from build123d import *

# Parameters (mm, degrees)
F0_R     = 1.778
F1_DEPTH = 5.08
F2_R     = 3.81
F2_R_2   = 1.778
F3_DEPTH = 6.35
F4_R     = 5.08
F5_R     = 1.016


with BuildPart() as f1:
    # F0 (on Front) → F1 (new body)
    with BuildSketch(Plane.XZ):
        with BuildLine():
            ThreePointArc((7.605604, -0.468175), (7.6164, -0.234198), (7.62, 0))
            ThreePointArc((7.62, 0), (7.6164, 0.234198), (7.605604, 0.468175))
            ThreePointArc((7.605604, 0.468175), (7.247051, 2.354709), (6.428249, 4.0917))
            ThreePointArc((6.428249, 4.0917), (6.164709, 4.478924), (5.877877, 4.849223))
            ThreePointArc((5.877877, 4.849223), (4.478924, 6.164709), (2.795522, 7.088685))
            ThreePointArc((2.795522, 7.088685), (2.354709, 7.247051), (1.905, 7.378033))
            ThreePointArc((1.905, 7.378033), (0, 7.62), (-1.905, 7.378033))
            ThreePointArc((-1.905, 7.378033), (-2.354709, 7.247051), (-2.795522, 7.088685))
            ThreePointArc((-2.795522, 7.088685), (-4.478924, 6.164709), (-5.877877, 4.849223))
            ThreePointArc((-5.877877, 4.849223), (-6.164709, 4.478924), (-6.428249, 4.0917))
            ThreePointArc((-6.428249, 4.0917), (-7.247051, 2.354709), (-7.605604, 0.468175))
            ThreePointArc((-7.605604, 0.468175), (-7.62, 0), (-7.605604, -0.468175))
            ThreePointArc((-7.605604, -0.468175), (-7.247051, -2.354709), (-6.428249, -4.0917))
            ThreePointArc((-6.428249, -4.0917), (-6.164709, -4.478924), (-5.877877, -4.849223))
            ThreePointArc((-5.877877, -4.849223), (-4.478924, -6.164709), (-2.795522, -7.088685))
            ThreePointArc((-2.795522, -7.088685), (-2.354709, -7.247051), (-1.905, -7.378033))
            ThreePointArc((-1.905, -7.378033), (0, -7.62), (1.905, -7.378033))
            ThreePointArc((1.905, -7.378033), (2.354709, -7.247051), (2.795522, -7.088685))
            ThreePointArc((2.795522, -7.088685), (4.478924, -6.164709), (5.877877, -4.849223))
            ThreePointArc((5.877877, -4.849223), (6.164709, -4.478924), (6.428249, -4.0917))
            ThreePointArc((6.428249, -4.0917), (7.247051, -2.354709), (7.605604, -0.468175))
        make_face()
        Circle(F0_R, mode=Mode.SUBTRACT)
        with BuildLine():
            ThreePointArc((6.428249, 4.0917), (7.247051, 2.354709), (7.605604, 0.468175))
            Line((7.605604, 0.468175), (9.689785, 1.412438))
            Line((9.689785, 1.412438), (11.830752, 3.04283))
            Line((11.830752, 3.04283), (11.35981, 4.49224))
            Line((11.35981, 4.49224), (8.66941, 4.552826))
            Line((8.66941, 4.552826), (6.428249, 4.0917))
        make_face()
        with BuildLine():
            Line((9.689785, -1.412438), (7.605604, -0.468175))
            ThreePointArc((7.605604, -0.468175), (7.247051, -2.354709), (6.428249, -4.0917))
            Line((6.428249, -4.0917), (8.66941, -4.552826))
            Line((8.66941, -4.552826), (11.35981, -4.49224))
            Line((11.35981, -4.49224), (11.830752, -3.04283))
            Line((11.830752, -3.04283), (9.689785, -1.412438))
        make_face()
        with BuildLine():
            ThreePointArc((2.795522, 7.088685), (4.478924, 6.164709), (5.877877, 4.849223))
            Line((5.877877, 4.849223), (7.00899, 6.838199))
            Line((7.00899, 6.838199), (7.782749, 9.415643))
            Line((7.782749, 9.415643), (6.549807, 10.311428))
            Line((6.549807, 10.311428), (4.337616, 8.779065))
            Line((4.337616, 8.779065), (2.795522, 7.088685))
        make_face()
        with BuildLine():
            Line((7.00899, -6.838199), (5.877877, -4.849223))
            ThreePointArc((5.877877, -4.849223), (4.478924, -6.164709), (2.795522, -7.088685))
            Line((2.795522, -7.088685), (4.337616, -8.779065))
            Line((4.337616, -8.779065), (6.549807, -10.311428))
            Line((6.549807, -10.311428), (7.782749, -9.415643))
            Line((7.782749, -9.415643), (7.00899, -6.838199))
        make_face()
        with BuildLine():
            ThreePointArc((-1.905, 7.378033), (0, 7.62), (1.905, 7.378033))
            Line((1.905, 7.378033), (1.651, 9.652))
            Line((1.651, 9.652), (0.762, 12.192))
            Line((0.762, 12.192), (-0.762, 12.192))
            Line((-0.762, 12.192), (-1.651, 9.652))
            Line((-1.651, 9.652), (-1.905, 7.378033))
        make_face()
        with BuildLine():
            Line((1.651, -9.652), (1.905, -7.378033))
            ThreePointArc((1.905, -7.378033), (0, -7.62), (-1.905, -7.378033))
            Line((-1.905, -7.378033), (-1.651, -9.652))
            Line((-1.651, -9.652), (-0.762, -12.192))
            Line((-0.762, -12.192), (0.762, -12.192))
            Line((0.762, -12.192), (1.651, -9.652))
        make_face()
        with BuildLine():
            ThreePointArc((-5.877877, 4.849223), (-4.478924, 6.164709), (-2.795522, 7.088685))
            Line((-2.795522, 7.088685), (-4.337616, 8.779065))
            Line((-4.337616, 8.779065), (-6.549807, 10.311428))
            Line((-6.549807, 10.311428), (-7.782749, 9.415643))
            Line((-7.782749, 9.415643), (-7.00899, 6.838199))
            Line((-7.00899, 6.838199), (-5.877877, 4.849223))
        make_face()
        with BuildLine():
            Line((-4.337616, -8.779065), (-2.795522, -7.088685))
            ThreePointArc((-2.795522, -7.088685), (-4.478924, -6.164709), (-5.877877, -4.849223))
            Line((-5.877877, -4.849223), (-7.00899, -6.838199))
            Line((-7.00899, -6.838199), (-7.782749, -9.415643))
            Line((-7.782749, -9.415643), (-6.549807, -10.311428))
            Line((-6.549807, -10.311428), (-4.337616, -8.779065))
        make_face()
        with BuildLine():
            ThreePointArc((-7.605604, 0.468175), (-7.247051, 2.354709), (-6.428249, 4.0917))
            Line((-6.428249, 4.0917), (-8.66941, 4.552826))
            Line((-8.66941, 4.552826), (-11.35981, 4.49224))
            Line((-11.35981, 4.49224), (-11.830752, 3.04283))
            Line((-11.830752, 3.04283), (-9.689785, 1.412438))
            Line((-9.689785, 1.412438), (-7.605604, 0.468175))
        make_face()
        with BuildLine():
            Line((-8.66941, -4.552826), (-6.428249, -4.0917))
            ThreePointArc((-6.428249, -4.0917), (-7.247051, -2.354709), (-7.605604, -0.468175))
            Line((-7.605604, -0.468175), (-9.689785, -1.412438))
            Line((-9.689785, -1.412438), (-11.830752, -3.04283))
            Line((-11.830752, -3.04283), (-11.35981, -4.49224))
            Line((-11.35981, -4.49224), (-8.66941, -4.552826))
        make_face()
    extrude(amount=F1_DEPTH)

    # F2 (on face) → F3 (join)
    with BuildSketch(Plane.XZ.offset(5.08)):
        Circle(F2_R)
        Circle(F2_R_2, mode=Mode.SUBTRACT)
    extrude(amount=F3_DEPTH)

    # F4
    f4_edges = [f1.edges().sort_by_distance(p)[0] for p in [
        (7.00899, -2.54, 6.838199),
        (4.337616, -2.54, 8.779065),
        (1.651, -2.54, 9.652),
        (-4.337616, -2.54, 8.779065),
        (-8.66941, -2.54, 4.552826),
        (-9.689785, -2.54, -1.412438),
        (-7.00899, -2.54, -6.838199),
        (-1.651, -2.54, -9.652),
        (4.337616, -2.54, -8.779065),
        (8.66941, -2.54, -4.552826),
        (9.689785, -2.54, 1.412438),
        (9.689785, -2.54, -1.412438),
        (8.66941, -2.54, 4.552826),
        (-1.651, -2.54, 9.652),
        (-7.00899, -2.54, 6.838199),
        (-9.689785, -2.54, 1.412438),
        (-8.66941, -2.54, -4.552826),
        (-4.337616, -2.54, -8.779065),
        (1.651, -2.54, -9.652),
        (7.00899, -2.54, -6.838199),
    ]]
    fillet(f4_edges, radius=F4_R)

    # F5
    f5_edges = [f1.edges().sort_by_distance(p)[0] for p in [
        (0.762, -2.54, 12.192),
        (-0.762, -2.54, 12.192),
        (-6.549807, -2.54, 10.311428),
        (-7.782749, -2.54, 9.415643),
        (-11.35981, -2.54, 4.49224),
        (6.549807, -2.54, 10.311428),
        (7.782749, -2.54, 9.415643),
        (11.35981, -2.54, 4.49224),
        (-11.830752, -2.54, 3.04283),
        (-11.830752, -2.54, -3.04283),
        (-11.35981, -2.54, -4.49224),
        (-7.782749, -2.54, -9.415643),
        (-6.549807, -2.54, -10.311428),
        (-0.762, -2.54, -12.192),
        (0.762, -2.54, -12.192),
        (6.549807, -2.54, -10.311428),
        (7.782749, -2.54, -9.415643),
        (11.830752, -2.54, -3.04283),
        (11.35981, -2.54, -4.49224),
        (11.830752, -2.54, 3.04283),
    ]]
    fillet(f5_edges, radius=F5_R)


solid = f1.part
Here's how the part is built. I have some questions about the finished solid (model axes, mm). A direction names the side the tool comes from. Coordinates: 2 decimals unless noted, no trailing zeros. Write each loop counter-clockwise with the first axis right and the second up, starting at its lowest first coordinate (ties: lowest second). Pieces come first, ordered by that corner, then holes. Notation, with made-up numbers: (68, 74) - (110, 74) arc R23 cw to (110, 86) - close; hole circle Ø9 at (-3.5, 43). An arc over 180 degrees is marked (long way). Use one line per item in the form item = value.
1) Suppose I cut it at D-D, the plane x = -4.25. Write out the boundary of the cut face in (y, z).
Solved:
outline = (-5.08, -8.66) - (0, -8.66) - (0, 8.66) - (-5.08, 8.66) - close
2) I need wall thicknesses on line 1 (X direction, y = -4, z = 7.75); line 2 (Y direction, x = 5.5, z = -9); line 3 (Z direction, x = 0, y = -8.25). Which ranges of each line are inside material? Lowest first, please.
Solved:
line_1 = -7.28 to -3.4, -1.86 to 1.86, 3.4 to 7.28
line_2 = -5.08 to 0
line_3 = -3.81 to -1.78, 1.78 to 3.81
3) Suppose I cut it at A-A, the plane x = 9.75. Write out the boundary of the cut face in (y, z), plus the area to 3 significant figures.
Solved:
outline = (-5.08, -4.53) - (0, -4.53) - (0, -1.49) - (-5.08, -1.49) - close; (-5.08, 1.49) - (0, 1.49) - (0, 4.53) - (-5.08, 4.53) - close
area = 30.9 mm2
4) Suppose I cut it at B-B, the plane z = -7.75. Write out the boundary of the cut face in (x, y), plus the area to 3 significant figures.
Solved:
outline = (-7.28, -5.08) - (-3.4, -5.08) - (-3.4, 0) - (-7.28, 0) - close; (-1.86, -5.08) - (1.86, -5.08) - (1.86, 0) - (-1.86, 0) - close; (3.4, -5.08) - (7.28, -5.08) - (7.28, 0) - (3.4, 0) - close
area = 58.4 mm2
5) Suppose I cut it at C-C, the plane y = -9. Write out the boundary of the cut face in (x, z).
Solved:
outline = circle Ø7.62 at (0, 0); hole circle Ø3.56 at (0, 0)
6) I'm going to push flat-ended pins straight in: P1, Ø3, axis at y = -1, z = -6.5, coming from the -X side; P2, Ø2, axis at y = -1, z = 1.5, coming from the +X side; P3, Ø1, axis at y = -4, z = 8.5, coming from the -X side. Where does each tip first touch, or does it pass through?
Solved:
P1 = -7.36
P2 = 11.12
P3 = -7.62
7) On a 3-axis mill with a long thin cutter (end or side, diameter ignored), from which of +Z, -Z, +X, -X, +Y, -Y can I reach the whole of each face in a straight line? I mean faces 4 (the cylindrical face through (-4.365, -2.576, 8.76)), 5 (the flat face through (7.38, -2.5, -8.07)), 6 (the cylindrical face through (-4.353, -2.576, -8.749)). Say none if no direction works.
Solved:
face_4 = +Z, +Y, -Y
face_5 = +X, +Y, -Y
face_6 = -Z, +Y, -Y
8) Thinking about a two-plate mould opening in X: for faces 1 (the flat face through (-7.279, -2.504, -4.267)), 2 (the flat face through (7.372, -2.504, 8.048)), 3 (the flat face through (-3, -5.08, 3)), which applies, released by +X, released by -X, zero draft, split by the parting line, or undercut?
Solved:
face_1 = undercut
face_2 = released by +X
face_3 = zero draft
